Design review of the part built by this model. Coordinates are the model's own, in mm. Face numbers are marked on the shaded views. A direction names the side the tool comes from. Give positions to 0.01 mm unless a question says otherwise; leave off trailing zeros. Write each loop counter-clockwise with the first axis right and the second up, starting at its lowest first coordinate (ties: lowest second). Pieces come first, ordered by that corner, then holes. Notation, with made-up numbers: (-6, -31.5) -> (16, -31.5) arc R23 ccw to (16, 0.5) -> close; hole circle Ø8 at (-24.5, 83.25). An arc over 180 degrees is marked (long way). Write each question's results on one line, items separated by ' | '. Start each with the question number.
(1) For the marked faces 1, 2, 3 and 4, list the 3-axis set-ups (+Z, -Z, +X, -X, +Y, -Y) from which the entire face can be reached by the end or side of a thin tool; tool diameter is ignored.
(2) Take a section at A-A (z = -4). State the section outline as (x, y) points, plus the area to 3 significant figures.
(3) To check wall thickness, follow probe 1 along Y at (x, z) = (2.5, -3); probe 2 along Z at (x, y) = (21, -1); probe 3 along Y at (x, z) = (35, -0.75). State the ranges of each line that lie inside material, in increasing order.
(4) Take a section at D-D (y = 18.5). State the section outline as (x, z) points.
(5) Take a section at B-B (y = 0). State the section outline as (x, z) points, plus the area to 3 significant figures.
(6) Clearance check with flat-ended pins moving along their axes: pin 1 (8 mm diameter, centred on x = 28.5, y = -0.5, fed in from +Z); pin 2 (15.5 mm diameter, centred on x = -4, y = -1, fed in from +Z); pin 3 (7 mm diameter, centred on x = 3.5, y = 2, fed in from -Z); pin 4 (7 mm diameter, centred on y = -1, z = -2.5, fed in from +X). State where each tip first meets the part, or that it passes through.
(7) Take a section at C-C (x = -16). State the section outline as (y, z) points.
from build123d import *

# Parameters (mm, degrees)
F0_W          = 49.99736
F0_H          = 13.9954
F1_DEPTH      = 5
F1_DEPTH_BACK = 5
F2_R          = 1
F3_R          = 10
F4_W          = 13.9954
F4_H          = 13.9954
F5_DEPTH      = 1
F5_DEPTH_BACK = 5
F6_T4_DEPTH   = 39.7122298797
F6_T9_DEPTH   = 39.7122298797
F7_SIZE       = 5
F8_W          = 7.0710678119
F8_H          = 13.9954
F9_DEPTH      = 25.4


# Not quite as in the source:
# - a fillet or chamfer that OpenCascade refuses, or shapes differently, is made with other operations: its cross-section is extruded or revolved along the edge and cut away or added


with BuildPart() as f1:
    # F0 (on Top) → F1 (new body, two sides)
    with BuildSketch(Plane.XY) as f1_sk:
        Rectangle(F0_W, F0_H)
    extrude(amount=F1_DEPTH)
    extrude(f1_sk.sketch, amount=-F1_DEPTH_BACK)

    # F2
    f2_edges = [f1.edges().sort_by_distance(p)[0] for p in [
        (-24.99868, 6.9977, 0),
    ]]
    fillet(f2_edges, radius=F2_R)

    # F3
    f3_edges = [f1.edges().sort_by_distance(p)[0] for p in [
        (-24.99868, -6.9977, 0),
    ]]
    fillet(f3_edges, radius=F3_R)

    # F4 (on face) → F5 (join, two sides)
    with BuildSketch(Plane.YZ.offset(24.99868)) as f5_sk:
        Rectangle(F4_W, F4_H)
    extrude(amount=F5_DEPTH)
    extrude(f5_sk.sketch, amount=-F5_DEPTH_BACK)

    # F6: chamfer of 5 on 2 edges, made by hand


with BuildPart() as f6_tool2:
    # F6_s3 → F6_t4 (new body)
    with BuildSketch(Plane.XZ.offset(-19.8561149398)):
        Polygon((19.99868, 1.9977), (24.99868, 6.9977), (19.99868, 6.9977), align=None)
    extrude(amount=F6_T4_DEPTH)

    split(bisect_by=Plane.XY.offset(5), keep=Keep.TOP)


with BuildPart() as f1_1:
    add(f1.part)

    # F6_t1: cut F6_tool2
    add(f6_tool2.part, mode=Mode.SUBTRACT)


with BuildPart() as f6_tool7:
    # F6_s8 → F6_t9 (new body)
    with BuildSketch(Plane.XZ.offset(19.8561149398)):
        Polygon((19.99868, -1.9977), (24.99868, -6.9977), (19.99868, -6.9977), align=None)
    extrude(amount=-F6_T9_DEPTH)

    split(bisect_by=Plane.XY.offset(-5), keep=Keep.BOTTOM)


with BuildPart() as f1_2:
    add(f1_1.part)

    # F6_t6: cut F6_tool7
    add(f6_tool7.part, mode=Mode.SUBTRACT)

    # F7
    f7_edges = [f1_2.edges().sort_by_distance(p)[0] for p in [
        (25.99868, 6.9977, 0),
    ]]
    chamfer(f7_edges, length=F7_SIZE)

    # F8 (on face) → F9 (join)
    with BuildSketch(Plane(origin=(13.99819, 13.99819, 0), x_dir=(-0.7071067812, 0.7071067812, 0), z_dir=(0.7071067812, 0.7071067812, 0))):
        with Locations((-13.4357218072, 0)):
            Rectangle(F8_W, F8_H)
    extrude(amount=F9_DEPTH)


solid = f1_2.part
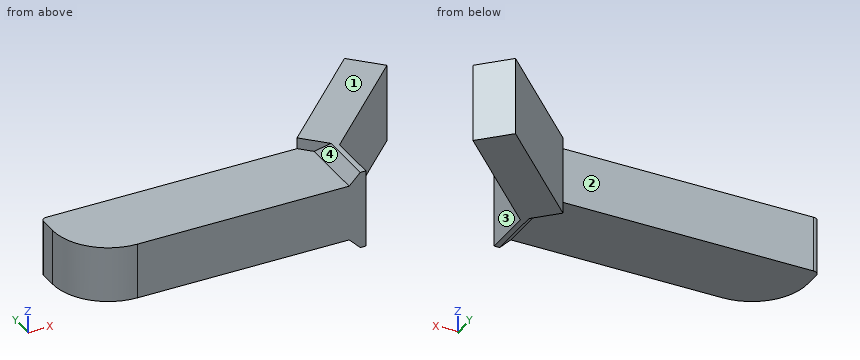
Report:
1) face 1: +Z, +X, -X, +Y, -Y | face 2: +Z, -Z, -X, +Y | face 3: +Z, -Z, +X, -Y | face 4: +Z, -X, -Y
2) outline: (-25, 3) arc R10 ccw to (-15, -7) -> (26, -7) -> (26, 2) -> (43.96, 19.96) -> (38.96, 24.96) -> (21, 7) -> (-24, 7) arc R1 ccw to (-25, 6) -> close | area: 859 mm2
3) probe 1: -7 to 7 | probe 2: -5 to 5 | probe 3: 11 to 21
4) outline: (32.5, -7) -> (42.5, -7) -> (42.5, 7) -> (32.5, 7) -> close
5) outline: (-24.54, -5) -> (23, -5) -> (25, -7) -> (26, -7) -> (26, 7) -> (25, 7) -> (23, 5) -> (-24.54, 5) -> close | area: 513 mm2
6) pin 1: z = 7 | pin 2: z = 5 | pin 3: z = -5 | pin 4: x = 26.5
7) outline: (-6.95, -5) -> (7, -5) -> (7, 5) -> (-6.95, 5) -> close
